from build123d import *

# Parameters (mm, degrees)
F0_W     = 127
F0_H     = 76.2
F1_DEPTH = 6.35
F2_T     = -5.08
F3_R     = 5.08
F4_R     = 5.08
F5_R     = 5.08
F6_R     = 5.08


with BuildPart() as f1:
    # F0 (on Top) → F1 (new body)
    with BuildSketch(Plane.XY):
        Rectangle(F0_W, F0_H)
    extrude(amount=F1_DEPTH)

    # F2
    f2_openings = [f1.faces().sort_by_distance(p)[0] for p in [
        (0, 0, 6.35),
    ]]
    offset(amount=F2_T, openings=f2_openings)

    # F3
    f3_edges = [f1.edges().sort_by_distance(p)[0] for p in [
        (58.42, 33.02, 5.715),
    ]]
    fillet(f3_edges, radius=F3_R)

    # F4
    f4_edges = [f1.edges().sort_by_distance(p)[0] for p in [
        (-58.42, 33.02, 5.715),
    ]]
    fillet(f4_edges, radius=F4_R)

    # F5
    f5_edges = [f1.edges().sort_by_distance(p)[0] for p in [
        (-58.42, -33.02, 5.715),
    ]]
    fillet(f5_edges, radius=F5_R)

    # F6
    f6_edges = [f1.edges().sort_by_distance(p)[0] for p in [
        (58.42, -33.02, 5.715),
    ]]
    fillet(f6_edges, radius=F6_R)


solid = f1.part
Could you check a few things on this model? Use its own coordinates, in mm. A direction names the side the tool comes from. Give positions to 0.01 mm unless a question says otherwise; leave off trailing zeros. Loops run counter-clockwise (first coordinate to the right, second up) from the corner with the lowest first, then second, coordinate; pieces in that order, holes last. Notation, with made-up numbers: (86.25, 25.25) -> (115.25, 25.25) arc R22 ccw to (115.25, 63.25) -> close; hole circle Ø4 at (-26, 88). An arc over 180 degrees is marked (long way). Answer as CSV lines item,"result". Start each with the question number.
(1) If we section it at B-B on y = 22: Write out the boundary of the cut face in (x, z), then the cut area to 3 significant figures.
(2) We'd pull the mould along X, two halves only. Please class faces 3 (the cylindrical face through (56.892, -31.571, 5.724)), 4 (the flat face through (63.5, -1, 3)), 5 (the flat face through (-5, -34, 6.35)): released by +X, released by -X, zero draft, split by the parting line, or undercut.
(3) Which directions (+Z, -Z, +X, -X, +Y, -Y) give clear straight access to the entire face, cutting with the end or side of a thin tool? Please do faces 1 (the cylindrical face through (-56.892, 31.571, 5.706)), 2 (the flat face through (-63.5, -1, 3)).
(4) I need wall thicknesses on probe 1 along Y at (x, z) = (31.5, 6); probe 2 along Z at (x, y) = (-55.5, 4.5). Which ranges of each line are inside material? Lowest first, please.
(5) If we section it at A-A on x = 15: Write out the boundary of the cut face in (y, z).
(6) I'm going to push a flat-ended pin straight in: pin 1 Ø8 at (x, y) = (28, -28.5) entering from +Z. Where does the tip first touch, or does it pass through?
Computed:
1,outline,"(-63.5, 0) -> (63.5, 0) -> (63.5, 6.35) -> (58.42, 6.35) -> (58.42, 5.08) -> (-58.42, 5.08) -> (-58.42, 6.35) -> (-63.5, 6.35) -> close"
1,area,"658 mm2"
2,face 3,"undercut"
2,face 4,"released by +X"
2,face 5,"zero draft"
3,face 1,"+Z"
3,face 2,"+Z, -Z, -X, +Y, -Y"
4,probe 1,"y = -38.1 to -33.02, 33.02 to 38.1"
4,probe 2,"z = 0 to 5.08"
5,outline,"(-38.1, 0) -> (38.1, 0) -> (38.1, 6.35) -> (33.02, 6.35) -> (33.02, 5.08) -> (-33.02, 5.08) -> (-33.02, 6.35) -> (-38.1, 6.35) -> close"
6,pin 1,"stops at z = 5.08"
